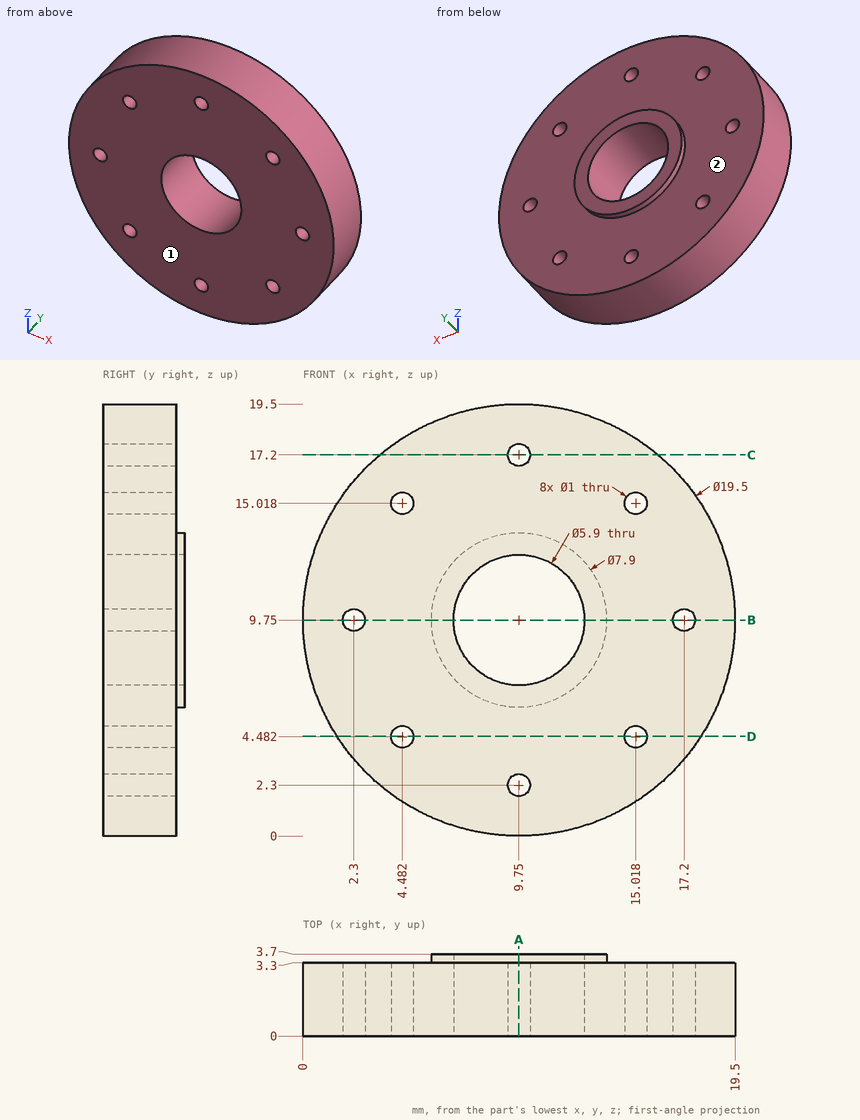
The drawing under review shows one solid part. Ordinate dimensions are in mm from its lowest x, y, z. A direction names the side the tool comes from. Coordinates: 2 decimals unless noted, no trailing zeros. Order: outer loops, then holes, each group sorted by start corner. A loop starts at its lowest first (then second) coordinate and runs counter-clockwise, first axis right, second up. Notation, with made-up numbers: (77.25, 17) -> (97.25, 17) arc R17 ccw to (97.25, 45) -> close; hole circle Ø4 at (31, 75). An arc over 180 degrees is marked (long way). Answer as CSV lines item,"result".
Q1. Wall thickness on line 1 along X through (y, z) = (1.65, 9.75); line 2 along X through (y, z) = (0.6, 15); line 3 along Z through (x, y) = (9.5, 1.65): over which ranges is each line inside the solid? List them lowest first. Write a range as [from, to].
Model answer:
line 1,"x = [0, 1.8], [2.8, 6.8], [12.7, 16.7], [17.7, 19.5]"
line 2,"x = [1.53, 3.98], [4.98, 14.52], [15.52, 17.97]"
line 3,"z = [0, 1.87], [2.73, 6.81], [12.69, 16.77], [17.63, 19.5]"
Q2. We need section C-C (z = 17.2). State the section outline as (x, y) points.
Model answer:
outline,"(3.46, 0) -> (9.25, 0) -> (9.25, 3.3) -> (3.46, 3.3) -> close; (10.25, 0) -> (16.04, 0) -> (16.04, 3.3) -> (10.25, 3.3) -> close"
Q3. For the marked faces 1 and 2, list the 3-axis set-ups (+Z, -Z, +X, -X, +Y, -Y) from which the entire face can be reached by the end or side of a thin tool; tool diameter is ignored.
Model answer:
face 1,"+Z, -Z, +X, -X, -Y"
face 2,"+Y"
Q4. Clearance check with a flat-ended pin moving along its axis: pin 1 Ø2 at (x, y) = (14.5, 1.5) entering from -Z. State where the tip first meets the part, or that it passes through.
Model answer:
pin 1,"stops at z = 0.75"
Q5. We need section B-B (z = 9.75). State the section outline as (x, y) points, plus the area to 3 significant figures.
Model answer:
outline,"(0, 0) -> (1.8, 0) -> (1.8, 3.3) -> (0, 3.3) -> close; (2.8, 0) -> (6.8, 0) -> (6.8, 3.7) -> (5.8, 3.7) -> (5.8, 3.3) -> (2.8, 3.3) -> close; (12.7, 0) -> (16.7, 0) -> (16.7, 3.3) -> (13.7, 3.3) -> (13.7, 3.7) -> (12.7, 3.7) -> close; (17.7, 0) -> (19.5, 0) -> (19.5, 3.3) -> (17.7, 3.3) -> close"
area,"39.1 mm2"
Q6. We need section A-A (x = 9.75). State the section outline as (y, z) points, plus the area to 3 significant figures.
Model answer:
outline,"(0, 0) -> (3.3, 0) -> (3.3, 1.8) -> (0, 1.8) -> close; (0, 2.8) -> (3.3, 2.8) -> (3.3, 5.8) -> (3.7, 5.8) -> (3.7, 6.8) -> (0, 6.8) -> close; (0, 12.7) -> (3.7, 12.7) -> (3.7, 13.7) -> (3.3, 13.7) -> (3.3, 16.7) -> (0, 16.7) -> close; (0, 17.7) -> (3.3, 17.7) -> (3.3, 19.5) -> (0, 19.5) -> close"
area,"39.1 mm2"
Q7. We need section D-D (z = 4.5). State the section outline as (x, y) points, plus the area to 3 significant figures.
Model answer:
outline,"(1.53, 0) -> (3.98, 0) -> (3.98, 3.3) -> (1.53, 3.3) -> close; (4.98, 0) -> (14.52, 0) -> (14.52, 3.3) -> (4.98, 3.3) -> close; (15.52, 0) -> (17.97, 0) -> (17.97, 3.3) -> (15.52, 3.3) -> close"
area,"47.6 mm2"
